Check sheet for the modelled part. Datum: model origin and axes. Units: mm. A direction names the side the tool comes from. Round coordinates to 2 decimals unless told otherwise and drop trailing zeros. Answer in a Markdown table with one row per item. Add a question column.
(1) Thickness scan on line 1 along X through (y, z) = (90, 6.5); line 2 along Z through (x, y) = (-10.75, 145.5); line 3 along Z through (x, y) = (11.5, 76). Record the ranges inside material, lowest first.
(2) Gauge pin test, flat ends, axial feed: pin 1 (4 mm diameter, centred on x = 0, y = 81.5, fed in from +Z); pin 2 (1 mm diameter, centred on y = 229, z = 1, fed in from -X); pin 3 (7 mm diameter, centred on x = -1, y = 200.5, fed in from +Z). Record the tip position at first contact, or that the pin passes through.
(3) Mould release check, pull along Y, two halves, no side actions. Record for faces 4 (the flat face through (0, 30, 3)), 5 (the cylindrical face through (0.29, 262.23, 0.49)), 6 (the flat face through (-10, 167, 3)): +Y half, -Y half, draft (parallel to the pull), parting line (faces both ways), or undercut.
(4) Cross-section at B-B on x = 0. Count the separate pieces of the cut face and the enclosed holes in it, then the cut area to 3 significant figures.
(5) Access from +Z, -Z, +X, -X, +Y, -Y to the whole of each face (thin tool, end or side, straight path). Record for faces 1 (the flat face through (10, 167, 3)), 2 (the flat face through (2, 138, 1)), 3 (the flat face through (0, 163, 4.1)).
from build123d import *

# Parameters (mm, degrees)
BOSS_EXTRUDE1_DEPTH                              = 270
CUT_EXTRUDE1_DEPTH                               = 271.477244884
F_0_4_0_4_DIAMETER_HOLE1_D                       = 0.4
CBORE_FOR_M4_HEX_HEAD_MACHINE_SCREW1_D           = 4.5
CBORE_FOR_M4_HEX_HEAD_MACHINE_SCREW1_DEPTH       = 4.1
CBORE_FOR_M4_HEX_HEAD_MACHINE_SCREW1_CBORE_D     = 8.5
CBORE_FOR_M4_HEX_HEAD_MACHINE_SCREW1_CBORE_DEPTH = 3.1
FILLET1_R                                        = 0.2
FILLET2_R                                        = 0.5
FILLET3_R                                        = 1
CUT_EXTRUDE2_REACH                               = 302.339
SKETCH7_R                                        = 2.5


with BuildPart() as part:
    # Sketch1 → Boss-Extrude1 (new body)
    with BuildSketch(Plane(origin=(0, 300, 0), x_dir=(1, 0, 0), z_dir=(0, 1, 0))):
        with BuildLine():
            Line((-13.5, -3), (-13.5, -8.7))
            Line((-13.5, -8.7), (13.5, -8.7))
            Line((13.5, -8.7), (13.5, -3))
            Line((13.5, -3), (7.8, -3))
            ThreePointArc((7.8, -3), (7.05, -2.25), (7.8, -1.5))
            Line((7.8, -1.5), (11, -1.5))
            Line((11, -1.5), (11, 0))
            Line((11, 0), (-11, 0))
            Line((-11, 0), (-11, -1.5))
            Line((-11, -1.5), (-7.8, -1.5))
            ThreePointArc((-7.8, -1.5), (-7.05, -2.25), (-7.8, -3))
            Line((-7.8, -3), (-13.5, -3))
        make_face()
    extrude(amount=-BOSS_EXTRUDE1_DEPTH)

    # Sketch2 → Cut-Extrude1 (cut, through all)
    with BuildSketch(Plane.XZ.offset(-30)):
        Polygon((8.75, 8.7), (-8.75, 8.7), (-8.75, 7.6), (-12, 7.6), (-12, 4.1), (12, 4.1), (12, 7.6), (8.75, 7.6), align=None)
    extrude(amount=-CUT_EXTRUDE1_DEPTH, mode=Mode.SUBTRACT)

    # Ø0.4 (0.4) Diameter Hole1 (through all)
    with Locations(Plane(origin=(0, 300, 0), x_dir=(1, 0, 0), z_dir=(0, 1, 0))):
        with Locations((-7.75, -4.1), (7.75, -4.1)):
            Hole(F_0_4_0_4_DIAMETER_HOLE1_D / 2)

    # CBORE for M4 Hex Head Machine Screw1
    with Locations(Plane.XY.offset(4.1)):
        with Locations((0, 260), (0, 200), (0, 140), (0, 80), (0, 20)):
            CounterBoreHole(CBORE_FOR_M4_HEX_HEAD_MACHINE_SCREW1_D / 2, CBORE_FOR_M4_HEX_HEAD_MACHINE_SCREW1_CBORE_D / 2, CBORE_FOR_M4_HEX_HEAD_MACHINE_SCREW1_CBORE_DEPTH, depth=CBORE_FOR_M4_HEX_HEAD_MACHINE_SCREW1_DEPTH)

    # Fillet1
    fillet1_edges = [part.edges().sort_by_distance(p)[0] for p in [
        (-11, 165, 1.5),
        (11, 165, 1.5),
    ]]
    fillet(fillet1_edges, radius=FILLET1_R)

    # Fillet2
    fillet2_edges = [part.edges().sort_by_distance(p)[0] for p in [
        (12, 165, 7.6),
        (12, 165, 4.1),
        (-12, 165, 4.1),
        (-12, 165, 7.6),
    ]]
    fillet(fillet2_edges, radius=FILLET2_R)

    # Fillet3
    fillet3_edges = [part.edges().sort_by_distance(p)[0] for p in [
        (13.5, 165, 3),
        (13.5, 165, 8.7),
        (-13.5, 165, 8.7),
        (-13.5, 165, 3),
    ]]
    fillet(fillet3_edges, radius=FILLET3_R)

    # Sketch7 → Cut-Extrude2 (cut, up to next)
    with BuildSketch(Plane.XY.offset(4.1), mode=Mode.PRIVATE) as cut_extrude2_sk1:
        with Locations((0, 290)):
            Circle(SKETCH7_R)
    cut_extrude2_tool1 = extrude(cut_extrude2_sk1.sketch, amount=-CUT_EXTRUDE2_REACH, mode=Mode.PRIVATE) & part.part
    # Sketch7 → Cut-Extrude2 (cut, up to next)
    with BuildSketch(Plane.XY.offset(4.1), mode=Mode.PRIVATE) as cut_extrude2_sk2:
        with Locations((0, 40)):
            Circle(SKETCH7_R)
    cut_extrude2_tool2 = extrude(cut_extrude2_sk2.sketch, amount=-CUT_EXTRUDE2_REACH, mode=Mode.PRIVATE) & part.part
    add(cut_extrude2_tool1.solids().sort_by_distance((0, 290, 4.1))[0], mode=Mode.SUBTRACT)
    add(cut_extrude2_tool2.solids().sort_by_distance((0, 40, 4.1))[0], mode=Mode.SUBTRACT)


solid = part.part
Answers:
| question | item | result |
|---|---|---|
| 1 | line 1 | x = -13.5 to -12, 12 to 13.5 |
| 1 | line 2 | z = 0 to 1.5, 3 to 4.1, 7.6 to 8.7 |
| 1 | line 3 | z = 3 to 4.1, 7.6 to 8.7 |
| 2 | pin 1 | stops at z = 1 |
| 2 | pin 2 | stops at x = -11 |
| 2 | pin 3 | stops at z = 4.1 |
| 3 | face 4 | -Y half |
| 3 | face 5 | undercut |
| 3 | face 6 | draft |
| 4 | separate pieces | 7 |
| 4 | enclosed holes | 0 |
| 4 | area | 943 mm^2 |
| 5 | face 1 | +X, +Y, -Y |
| 5 | face 2 | +Z |
| 5 | face 3 | +Z, +Y, -Y |
